Geometry check sheet. Reference: the model listing, model coordinates, mm. A direction names the side the tool comes from. Give positions to 0.01 mm unless a question says otherwise; leave off trailing zeros. Order: outer loops, then holes, each group sorted by start corner. A loop starts at its lowest first (then second) coordinate and runs counter-clockwise, first axis right, second up. Notation, with made-up numbers: M 34.25,52 L 57.25,52 A20 cw 57.25,85 Z; hole C -27.75,-25.5 d5. An arc over 180 degrees is marked long. Answer as CSV lines item,"result". Start each with the question number.
Autodesk Inventor part; units mm, degrees
ref_plane "YZ Plane" through (0, 0, 0) normal (1, 0, 0) x (0, 1, 0)
ref_plane "XZ Plane" through (0, 0, 0) normal (0, 1, 0) x (-1, 0, 0)
ref_plane "XY Plane" through (0, 0, 0) normal (0, 0, 1) x (1, 0, 0)
sketch "Sketch1" plane through (0, 0, 0) normal (0, 0, 1) x (1, 0, 0)
  line L0 (-35.3228, 16.049) -> (-9.9228, 16.049)
  line L1 (-9.9228, 16.049) -> (-9.9228, -34.751)
  line L2 (-9.9228, -34.751) -> (-35.3228, -34.751)
  line L3 (-35.3228, -34.751) -> (-35.3228, 16.049)
  line L4 (-13.0978, 12.874) -> (-32.1478, 12.874)
  line L5 (-32.1478, 12.874) -> (-32.1478, -31.576)
  line L6 (-32.1478, -31.576) -> (-13.0978, -31.576)
  line L7 (-13.0978, -31.576) -> (-13.0978, 12.874)
  point P0 (0, 0)
  dimension "d0" = 25.4
  dimension "d1" = 50.8
  dimension "d2" = 3.175
extrude "Extrusion1" add sketch "Sketch1" along normal blind 1008.38
sketch "Sketch2" plane through (-35.3228, -34.751, 0) normal (-1, 0, 0) x (0, 0, 1)
  line L0 (0, 0) -> (0, 50.8) construction
  line L1 (0, 25.4) -> (25.4, 25.4) construction
  circle A0 centre (25.4, 25.4) radius 12.7
  point P0 (0, 34.751)
  dimension "d5" = 25.4
  dimension "d9" = 25.4
extrude "Extrusion2" cut sketch "Sketch2" against normal blind 254
sketch "Sketch3" plane through (-35.3228, -34.751, 0) normal (-1, 0, 0) x (0, 0, 1)
  line L0 (0, 50.8) -> (1008.38, 50.8) construction
  line L1 (0, 50.8) -> (0, 46.0248) construction
  line L2 (0, 0) -> (0, 50.8) construction
  line L3 (0, 46.0248) -> (13.4874, 46.0248) construction
  line L4 (13.4874, 46.0248) -> (37.3126, 46.0248) construction
  line L5 (13.4874, 46.0248) -> (13.4874, 4.7752) construction
  line L6 (37.3126, 46.0248) -> (37.3126, 4.7752) construction
  circle A0 centre (13.4874, 4.7752) radius 2.5797
  circle A1 centre (37.3126, 4.7752) radius 2.5797
  circle A2 centre (37.3126, 46.0248) radius 2.5797
  circle A3 centre (13.4874, 46.0248) radius 2.5797
  point P0 (0, 34.751)
  dimension "d10" = 4.7752
  dimension "d11" = 13.4874
  dimension "d12" = 23.8252
  dimension "d13" = 41.2496
  dimension "d14" = 41.2496
  dimension "d15" = 5.1594
  dimension "d16" = 5.1594
  dimension "d17" = 5.1594
  dimension "d18" = 5.1594
extrude "Extrusion3" cut sketch "Sketch3" against normal blind 25.4
properties part number "34.48in Arm Bea"
Item 1: Access from +Z, -Z, +X, -X, +Y, -Y to the whole of each face (thin tool, end or side, straight path). Record for faces 1 (the face through (-22, -34.751, 497)), 2 (the face through (-22, 12.874, 25)).
Item 2: Scan lines: line 1 along X through (y, z) = (-31.5, 258.5); line 2 along Y through (x, z) = (-13.75, 891.5); line 3 along Y through (x, z) = (-33.35, 25.4). Record each from-to range of solid material in increasing order.
Item 3: Draft check along X on faces 3 (the face through (-9.923, -9, 497)), 4 (the face through (-13.098, -10, 497)), 5 (the face through (-35.323, -10, 497)). Enter one of: pulls with the +X half, pulls with the -X half, needs draft (parallel to the pull), parting line crosses it, or undercut.
Item 4: Section check A-A on x = -22.5. Record the boundary of the cut face in (y, z), then the cut area to 3 significant figures.
Item 5: Depth check by flat-ended pin: pin 1 Ø4 at (y, z) = (11.27, 37.31) entering from -X. Enter the tip coordinate at first touch or a pass-through.
Item 6: Section check B-B on z = 25.4. Record the boundary of the cut face in (x, y), then the cut area to 3 significant figures.
Item 7: Section check C-C on z = 669. Record the boundary of the cut face in (x, y), then the cut area to 3 significant figures.
Numbers:
1,face 1,"+Z, -Z, +X, -X, -Y"
1,face 2,"+Z, -Z"
2,line 1,"-35.32 to -32.15, -13.1 to -9.92"
2,line 2,"-34.75 to -31.58, 12.87 to 16.05"
2,line 3,"-34.75 to -22.05, 3.35 to 16.05"
3,face 3,"pulls with the +X half"
3,face 4,"undercut"
3,face 5,"pulls with the -X half"
4,outline,"M -34.75,0 L -31.58,0 L -31.58,11.46 A2.58 cw -31.58,15.51 L -31.58,35.29 A2.58 cw -31.58,39.34 L -31.58,1008.38 L -34.75,1008.38 Z; M 12.87,0 L 16.05,0 L 16.05,1008.38 L 12.87,1008.38 L 12.87,39.34 A2.58 cw 12.87,35.29 L 12.87,15.51 A2.58 cw 12.87,11.46 Z"
4,area,"6,390 mm2"
5,pin 1,"through"
6,outline,"M -35.32,-34.75 L -9.92,-34.75 L -9.92,-22.05 L -13.1,-22.05 L -13.1,-31.58 L -32.15,-31.58 L -32.15,-22.05 L -35.32,-22.05 Z; M -35.32,3.35 L -32.15,3.35 L -32.15,12.87 L -13.1,12.87 L -13.1,3.35 L -9.92,3.35 L -9.92,16.05 L -35.32,16.05 Z"
6,area,"282 mm2"
7,outline,"M -35.32,-34.75 L -9.92,-34.75 L -9.92,16.05 L -35.32,16.05 Z; hole M -32.15,-31.58 L -13.1,-31.58 L -13.1,12.87 L -32.15,12.87 Z"
7,area,"444 mm2"
